Verification items for the finished model (mm, model axes). Face numbers are marked on the shaded views. A direction names the side the tool comes from. Round coordinates to 2 decimals unless told otherwise and drop trailing zeros. Write each loop counter-clockwise with the first axis right and the second up, starting at its lowest first coordinate (ties: lowest second). Pieces come first, ordered by that corner, then holes. Notation, with made-up numbers: M 11.5,-38.75 L 16.5,-38.75 A16 ccw 16.5,-33.75 Z; hole C 82.25,-21.5 d3. An arc over 180 degrees is marked long. Answer in a Markdown table with one row per item. Add a question column.
1. Sectioned sample at A-A on z = 1.5. Record the cut outline in (x, y).
2. Sectioned sample at B-B on x = 42.79. Record the cut outline in (y, z).
3. Sectioned sample at D-D on z = 17.75. Record the cut outline in (x, y), plus the area to 3 significant figures.
4. Sectioned sample at C-C on y = 56.5. Record the cut outline in (x, z), plus the area to 3 significant figures.
5. Material ranges on probe 1 along X at (y, z) = (4.5, 3); probe 2 along Y at (x, z) = (42.79, 8); probe 3 along Y at (x, z) = (41, 7.5), recorded low to high.
6. Set-up check for the marked faces 4, 5 and 6: record each of +Z, -Z, +X, -X, +Y, -Y from which the full face is reachable in a straight line by a thin tool's end or side.
7. Go/stop test with flat-tipped pins: pin 1 Ø0.6 at (x, y) = (24, 58.5) entering from +Z; pin 2 Ø10 at (x, y) = (16.5, 64.5) entering from +Z; pin 3 Ø8 at (x, z) = (29.5, 9.5) entering from +Y. Record where each tip stops, or that it passes through.
8. Draft check along X on the marked faces 1, 2 and 3. Enter one of: pulls with the +X half, pulls with the -X half, needs draft (parallel to the pull), parting line crosses it, or undercut.
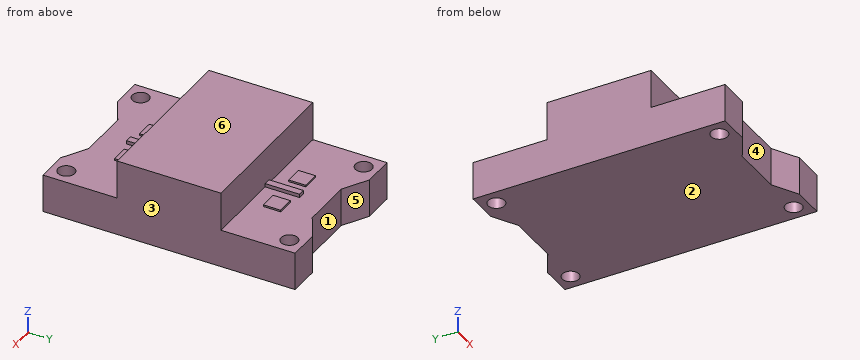
Autodesk Fusion 360 part; units mm, degrees
sketch "Sketch1" plane through (0, 0, 0) normal (0, 0, 1) x (1, 0, 0)
  line L0 (47.3, 0) -> (47.3, 72.8)
  line L1 (0, 72.8) -> (0, 0)
  circle A0 centre (4.51, 4.21) radius 2.41
  line L2 (0, 36.4) -> (47.3, 36.4) construction
  line L3 (0, 21.4) -> (47.3, 21.4)
  line L4 (23.65, 72.8) -> (23.65, -0.0931) construction
  line L5 (16.2, 4.1569) -> (31.1, 4.1569)
  line L6 (16.2, 4.1569) -> (9, 0)
  line L7 (31.1, 4.1569) -> (38.3, 0)
  circle A1 centre (42.79, 4.21) radius 2.41
  line L8 (0, 0) -> (9, 0)
  line L9 (38.3, 0) -> (47.3, 0)
  line L10 (0, 72.8) -> (47.3, 72.8) construction
  line L11 (22.65, 21.4) -> (24.65, 21.4)
  line L12 (24.65, 21.4) -> (24.65, 11.4)
  line L13 (24.65, 11.4) -> (22.65, 11.4)
  line L14 (22.65, 11.4) -> (22.65, 21.4)
  line L15 (19.65, 17.4) -> (14.65, 17.4)
  line L16 (14.65, 17.4) -> (14.65, 12.4)
  line L17 (14.65, 12.4) -> (19.65, 12.4)
  line L18 (19.65, 12.4) -> (19.65, 17.4)
  line L19 (32.65, 12.4) -> (27.65, 12.4)
  line L20 (27.65, 12.4) -> (27.65, 17.4)
  line L21 (32.65, 17.4) -> (32.65, 12.4)
  line L22 (27.65, 17.4) -> (32.65, 17.4)
  line L23 (16.2, 68.6431) -> (31.1, 68.6431)
  line L24 (14.65, 55.4) -> (14.65, 60.4)
  line L25 (38.3, 72.8) -> (47.3, 72.8)
  line L26 (24.65, 51.4) -> (24.65, 61.4)
  line L27 (27.65, 60.4) -> (27.65, 55.4)
  line L28 (22.65, 61.4) -> (22.65, 51.4)
  line L29 (16.2, 68.6431) -> (9, 72.8)
  line L30 (19.65, 60.4) -> (19.65, 55.4)
  line L31 (32.65, 60.4) -> (27.65, 60.4)
  line L32 (31.1, 68.6431) -> (38.3, 72.8)
  line L33 (19.65, 55.4) -> (14.65, 55.4)
  line L34 (14.65, 60.4) -> (19.65, 60.4)
  line L35 (24.65, 61.4) -> (22.65, 61.4)
  circle A2 centre (42.79, 68.59) radius 2.41
  line L36 (32.65, 55.4) -> (32.65, 60.4)
  line L37 (0, 72.8) -> (9, 72.8)
  line L38 (23.65, 0) -> (23.65, 72.8931) construction
  line L39 (27.65, 55.4) -> (32.65, 55.4)
  circle A3 centre (4.51, 68.59) radius 2.41
  line L40 (0, 51.4) -> (47.3, 51.4)
  point P0 (23.65, 4.1569)
  point P1 (23.65, 21.4)
  point P2 (0, 72.8)
  point P3 (23.65, 68.6431)
  dimension "d1" = 47.3
  dimension "d2" = 72.8
  dimension "d3" = 4.82
  dimension "d4" = 4.51
  dimension "d5" = 4.21
  dimension "d6" = 15
  dimension "d7" = 16.2
  dimension "d8" = 4.25
  dimension "d9" = 30
  dimension "d10" = 9
  dimension "d11" = 2
  dimension "d12" = 10
  dimension "d13" = 5
  dimension "d14" = 5
  dimension "d15" = 4
  dimension "d16" = 4
extrude "Extrude1" add sketch "Sketch1" along normal blind 22.2 contours L0 L1 L3 L11 L40
extrude "Extrude2" add sketch "Sketch1" along normal blind 12 contours L3 L11 L12 L13 L14 | L26 L28 L35 L40
extrude "Extrude3" add sketch "Sketch1" along normal blind 11 contours L0 L1 L3 L5 L6 L7 L8 L9 L12 L13 L14 | L0 L1 L23 L25 L26 L28 L29 L32 L35 L37 L40
extrude "Extrude4" add sketch "Sketch1" along normal blind 11.5 contours L15 L16 L17 L18 | L19 L20 L21 L22 | L24 L30 L33 L34 | L27 L31 L36 L39
equation "d4 = ( 4.82 / 2 ) * 1 mm + 2.1 mm"
equation "d5 = ( 4.82 / 2 ) * 1 mm + 1.8 mm"
Geometry check:
| question | item | result |
|---|---|---|
| 1 | outline | M 0,0 L 9,0 L 16.2,4.16 L 31.1,4.16 L 38.3,0 L 47.3,0 L 47.3,72.8 L 38.3,72.8 L 31.1,68.64 L 16.2,68.64 L 9,72.8 L 0,72.8 Z; hole C 4.51,4.21 d4.82; hole C 4.51,68.59 d4.82; hole C 42.79,4.21 d4.82; hole C 42.79,68.59 d4.82 |
| 2 | outline | M 0,0 L 1.8,0 L 1.8,11 L 0,11 Z; M 6.62,0 L 66.18,0 L 66.18,11 L 51.4,11 L 51.4,22.2 L 21.4,22.2 L 21.4,11 L 6.62,11 Z; M 71,0 L 72.8,0 L 72.8,11 L 71,11 Z |
| 3 | outline | M 0,21.4 L 47.3,21.4 L 47.3,51.4 L 0,51.4 Z |
| 3 | area | 1,420 mm2 |
| 4 | outline | M 0,0 L 47.3,0 L 47.3,11 L 32.65,11 L 32.65,11.5 L 27.65,11.5 L 27.65,11 L 24.65,11 L 24.65,12 L 22.65,12 L 22.65,11 L 19.65,11 L 19.65,11.5 L 14.65,11.5 L 14.65,11 L 0,11 Z |
| 4 | area | 527 mm2 |
| 5 | probe 1 | x = 0 to 2.12, 6.9 to 40.4, 45.18 to 47.3 |
| 5 | probe 2 | y = 0 to 1.8, 6.62 to 66.18, 71 to 72.8 |
| 5 | probe 3 | y = 0 to 2.6, 5.82 to 66.98, 70.2 to 72.8 |
| 6 | face 4 | +Z, -Z, -Y |
| 6 | face 5 | +Z, -Z, +Y |
| 6 | face 6 | +Z, +X, -X, +Y, -Y |
| 7 | pin 1 | stops at z = 12 |
| 7 | pin 2 | stops at z = 11.5 |
| 7 | pin 3 | stops at y = 70.03 |
| 8 | face 1 | undercut |
| 8 | face 2 | needs draft |
| 8 | face 3 | pulls with the +X half |
